from build123d import *

# Parameters (mm, degrees)
BOSS_EXTRUDE1_DEPTH = 250
BOSS_EXTRUDE6_DEPTH = 125
BOSS_EXTRUDE7_DEPTH = 125
BOSS_EXTRUDE8_DEPTH = 30


with BuildPart() as part:
    # Sketch1 → Boss-Extrude1 (new body)
    with BuildSketch(Plane(origin=(0, 0, 0), x_dir=(0, 0, -1), z_dir=(1, 0, 0))):
        with BuildLine():
            Line((-10, 7.5), (10, 7.5))
            ThreePointArc((10, 7.5), (17.5, 0), (10, -7.5))
            Line((10, -7.5), (-10, -7.5))
            ThreePointArc((-10, -7.5), (-17.5, 0), (-10, 7.5))
        make_face()
    extrude(amount=BOSS_EXTRUDE1_DEPTH)

    # Sketch11 → Boss-Extrude6 (add)
    with BuildSketch(Plane(origin=(0, 7.5, 0), x_dir=(1, 0, 0), z_dir=(0, 1, 0))):
        with BuildLine():
            Line((1.220843579, -10), (1.220843579, 10))
            ThreePointArc((1.220843579, 10), (8.447072594, 17.226229015), (15.673301609, 10))
            Line((15.673301609, 10), (15.673301609, -10))
            ThreePointArc((15.673301609, -10), (8.447072594, -17.226229015), (1.220843579, -10))
        make_face()
    extrude(amount=BOSS_EXTRUDE6_DEPTH)

    # Sketch12 → Boss-Extrude7 (add)
    with BuildSketch(Plane(origin=(-58.413349195, 58.413349195, 0), x_dir=(-0.7071067811865476, -0.7071067811865476, 0), z_dir=(0.7071067811865476, -0.7071067811865476, 0))):
        with BuildLine():
            Line((-105.56811993, -15), (-105.56811993, 15))
            ThreePointArc((-105.56811993, 15), (-100.022563681, 20.545556249), (-94.477007433, 15))
            Line((-94.477007433, 15), (-94.477007433, -15))
            ThreePointArc((-94.477007433, -15), (-100.022563681, -20.545556249), (-105.56811993, -15))
        make_face()
    extrude(amount=-BOSS_EXTRUDE7_DEPTH)

    # Sketch13 → Boss-Extrude8 (add)
    with BuildSketch(Plane(origin=(0, 0, 15), x_dir=(0.7071067811865476, -0.7071067811865476, 0), z_dir=(0, 0, 1))):
        with BuildLine():
            Line((-207.608950656, 105.56811993), (-203.079358094, 105.56811993))
            ThreePointArc((-203.079358094, 105.56811993), (-205.344154375, 106.506229266), (-207.608950656, 105.56811993))
        make_face()
        with BuildLine():
            Line((-200.108950656, 105.56811993), (-195.579358094, 105.56811993))
            ThreePointArc((-195.579358094, 105.56811993), (-197.844154375, 106.506229266), (-200.108950656, 105.56811993))
        make_face()
        with BuildLine():
            Line((-192.608950656, 105.56811993), (-188.079358094, 105.56811993))
            ThreePointArc((-188.079358094, 105.56811993), (-190.344154375, 106.506229266), (-192.608950656, 105.56811993))
        make_face()
        with BuildLine():
            Line((-185.108950656, 105.56811993), (-180.579358094, 105.56811993))
            ThreePointArc((-180.579358094, 105.56811993), (-182.844154375, 106.506229266), (-185.108950656, 105.56811993))
        make_face()
        with BuildLine():
            Line((-177.608950656, 105.56811993), (-173.079358094, 105.56811993))
            ThreePointArc((-173.079358094, 105.56811993), (-175.344154375, 106.506229266), (-177.608950656, 105.56811993))
        make_face()
        with BuildLine():
            Line((-170.108950656, 105.56811993), (-165.579358094, 105.56811993))
            ThreePointArc((-165.579358094, 105.56811993), (-167.844154375, 106.506229266), (-170.108950656, 105.56811993))
        make_face()
        with BuildLine():
            Line((-162.608950656, 105.56811993), (-158.079358094, 105.56811993))
            ThreePointArc((-158.079358094, 105.56811993), (-160.344154375, 106.506229266), (-162.608950656, 105.56811993))
        make_face()
        with BuildLine():
            Line((-155.108950656, 105.56811993), (-150.579358094, 105.56811993))
            ThreePointArc((-150.579358094, 105.56811993), (-152.844154375, 106.506229266), (-155.108950656, 105.56811993))
        make_face()
        with BuildLine():
            Line((-147.608950656, 105.56811993), (-143.079358094, 105.56811993))
            ThreePointArc((-143.079358094, 105.56811993), (-145.344154375, 106.506229266), (-147.608950656, 105.56811993))
        make_face()
        with BuildLine():
            Line((-140.108950656, 105.56811993), (-135.579358094, 105.56811993))
            ThreePointArc((-135.579358094, 105.56811993), (-137.844154375, 106.506229266), (-140.108950656, 105.56811993))
        make_face()
        with BuildLine():
            Line((-132.608950656, 105.56811993), (-128.079358094, 105.56811993))
            ThreePointArc((-128.079358094, 105.56811993), (-130.344154375, 106.506229266), (-132.608950656, 105.56811993))
        make_face()
        with BuildLine():
            Line((-125.108950656, 105.56811993), (-120.579358094, 105.56811993))
            ThreePointArc((-120.579358094, 105.56811993), (-122.844154375, 106.506229266), (-125.108950656, 105.56811993))
        make_face()
        with BuildLine():
            Line((-117.608950656, 105.56811993), (-113.079358094, 105.56811993))
            ThreePointArc((-113.079358094, 105.56811993), (-115.344154375, 106.506229266), (-117.608950656, 105.56811993))
        make_face()
        with BuildLine():
            Line((-110.108950656, 105.56811993), (-105.579358094, 105.56811993))
            ThreePointArc((-105.579358094, 105.56811993), (-107.844154375, 106.506229266), (-110.108950656, 105.56811993))
        make_face()
        with BuildLine():
            Line((-102.608950656, 105.56811993), (-98.079358094, 105.56811993))
            ThreePointArc((-98.079358094, 105.56811993), (-100.344154375, 106.506229266), (-102.608950656, 105.56811993))
        make_face()
        with BuildLine():
            Line((-95.108950656, 105.56811993), (-90.579358094, 105.56811993))
            ThreePointArc((-90.579358094, 105.56811993), (-92.844154375, 106.506229266), (-95.108950656, 105.56811993))
        make_face()
        with BuildLine():
            Line((-87.608950656, 105.56811993), (-83.079358094, 105.56811993))
            ThreePointArc((-83.079358094, 105.56811993), (-85.344154375, 106.506229266), (-87.608950656, 105.56811993))
        make_face()
    extrude(amount=-BOSS_EXTRUDE8_DEPTH)


solid = part.part
Could you check a few things on this model? Use its own coordinates, in mm. A direction names the side the tool comes from. Round coordinates to 2 decimals unless told otherwise and drop trailing zeros. Order: outer loops, then holes, each group sorted by start corner. A loop starts at its lowest first (then second) coordinate and runs counter-clockwise, first axis right, second up.
Q1. Imagine slicing it at A-A, the plane y = 0. List the corners of the cut face in (x, z) for me.
Geometry says:
outline: (0, -17.5) - (250, -17.5) - (250, 17.5) - (0, 17.5) - close
Q2. Imagine slicing it at B-B, the plane x = 108. List the corners of the cut face in (y, z) for me, then the cut area to 3 significant figures.
Geometry says:
outline: (-7.5, -10) arc R7.5 ccw to (7.5, -10) - (7.5, 10) arc R7.5 ccw to (-7.5, 10) - close
area: 477 mm2
Q3. Please list where these lines run through material, in increasing order: probe 1 along Y at (x, z) = (141.5, -9); probe 2 along X at (y, z) = (130, -3.5); probe 3 along Y at (x, z) = (121.5, -14.5).
Geometry says:
probe 1: y = -7.5 to 7.5
probe 2: x = 1.22 to 15.67
probe 3: y = -6 to 6
Q4. I'm going to push flat-ended pins straight in: P1, Ø8, axis at x = 203, z = -14.5, coming from the -Y side; P2, Ø8, axis at y = 84, z = -2, coming from the -X side; P3, Ø3.5, axis at x = -27.5, y = 177, coming from the -Z side. Where does each tip first touch, or does it pass through?
Geometry says:
P1: stops at y = -7.48
P2: stops at x = 1.22
P3: stops at z = -18.9
Q5. Thinking about a two-plate mould opening in Y: for faces 1 (the face through (8.288, 69.125, -17.224)), 2 (the face through (9, 7.5, 13)), 3 (the face through (-76.13, 217.473, -0.288)), 4 (the face through (0, 0, 0)), which applies, released by +Y, released by -Y, zero draft, split by the parting line, or undercut?
Geometry says:
face 1: undercut
face 2: undercut
face 3: released by +Y
face 4: zero draft
Q6. Which directions (+Z, -Z, +X, -X, +Y, -Y) give clear straight access to the entire face, cutting with the end or side of a thin tool? Please do faces 5 (the face through (15.8, 132.626, -0.096)), 6 (the face through (15.673, 69, 0)), 7 (the face through (1.221, 69, 0)).
Geometry says:
face 5: +X
face 6: +Z, -Z, +X
face 7: +Z, -Z, -X
